Read the model definition and answer for the solid it produces. Units are mm, in the model's axes. Give positions to 0.01 mm unless a question says otherwise; leave off trailing zeros. Write each loop counter-clockwise with the first axis right and the second up, starting at its lowest first coordinate (ties: lowest second). Pieces come first, ordered by that corner, then holes. Notation, with made-up numbers: (17.5, 54) -> (38.5, 54) arc R8 ccw to (38.5, 65) -> close; hole circle Ø1 at (40, -4). An arc over 180 degrees is marked (long way). Answer as CSV lines item,"result". Start each with the question number.
1. The part is cut by section B-B, the plane x = 47. Determine the outline of the cut face in (y, z), and give its area (3 significant figures).
2. The part is cut by section A-A, the plane z = -244. Determine the outline of the cut face in (x, y), and give its area (3 significant figures).
3. The part is cut by section C-C, the plane x = 257. Determine the outline of the cut face in (y, z).
4. Find the intervals of material crossed by line 1 (X direction, y = 3.25, z = -40); line 2 (Z direction, x = 102.5, y = 2.5); line 3 (Z direction, x = 187, y = 3.25), in increasing order.
5. The part is cut by section D-D, the plane y = 4. Give the number of separate pieces and of enclosed holes in the cut face, and give its area (3 significant figures).
6. Given pin 1 (1.8 mm diameter, centred on x = 144.5, y = 2, fed in from -Z); pin 2 (1.5 mm diameter, centred on x = 162.5, y = 2.5, fed in from -Z); pin 3 (1.8 mm diameter, centred on x = 153.5, y = 2.5, fed in from +Z), each flat-ended and moving along its own axis, determine where each tip first touches the part or whether it passes through.
from build123d import *

# Parameters (mm, degrees)
SUPPORT_DEPTH = 6
SKETCH2_W     = 60
SKETCH2_H     = 100
LITE_DEPTH    = 468.118828565
FILLET1_R     = 1
FILLET2_R     = 1
SKETCH3_W     = 6
SKETCH3_H     = 40
SKETCH3_W_2   = 40
SKETCH3_H_2   = 6
MOUNT_DEPTH   = 468.118828565


with BuildPart() as part:
    # Sketch1 → support (new body)
    with BuildSketch(Plane(origin=(0, 0, 0), x_dir=(1, 0, 0), z_dir=(0, 1, 0))):
        Polygon((300, 0), (300, -12), (180, -70), (174, -70), (0, -6), (0, 0), (0, 288), (0, 294), (174, 358), (180, 358), (300, 300), (300, 288), align=None)
    extrude(amount=SUPPORT_DEPTH)

    # Sketch2 → lite (cut, through all)
    with BuildSketch(Plane(origin=(0, 6, 0), x_dir=(1, 0, 0), z_dir=(0, 1, 0))):
        Polygon((95.999022376, -20), (164.988314579, -20), (164.988314579, -45.375371845), align=None)
        Polygon((184.988314579, -20), (184.988314579, -45.375371845), (237.489083913, -20), align=None)
        Polygon((95.999022376, 308), (164.988314579, 333.375371845), (164.988314579, 308), align=None)
        Polygon((184.988314579, 333.375371845), (237.489083913, 308), (184.988314579, 308), align=None)
        with Locations((245, 64)):
            Rectangle(SKETCH2_W, SKETCH2_H)
        with Locations((150, 64)):
            Rectangle(SKETCH2_W, SKETCH2_H)
        with Locations((55, 64)):
            Rectangle(SKETCH2_W, SKETCH2_H)
        with Locations((55, 224)):
            Rectangle(SKETCH2_W, SKETCH2_H)
        with Locations((150, 224)):
            Rectangle(SKETCH2_W, SKETCH2_H)
        with Locations((245, 224)):
            Rectangle(SKETCH2_W, SKETCH2_H)
    extrude(amount=-LITE_DEPTH, mode=Mode.SUBTRACT)

    # Fillet1
    fillet1_edges = [part.edges().sort_by_distance(p)[0] for p in [
        (0, 3, -294),
        (174, 3, -358),
        (180, 3, -358),
        (300, 3, -300),
        (300, 3, 12),
        (180, 3, 70),
        (174, 3, 70),
        (0, 3, 6),
    ]]
    fillet(fillet1_edges, radius=FILLET1_R)

    # Fillet2
    fillet2_edges = [part.edges().sort_by_distance(p)[0] for p in [
        (85, 3, -114),
        (85, 3, -14),
        (25, 3, -14),
        (25, 3, -114),
        (85, 3, -274),
        (85, 3, -174),
        (25, 3, -174),
        (25, 3, -274),
        (180, 3, -274),
        (180, 3, -174),
        (120, 3, -174),
        (120, 3, -274),
        (275, 3, -274),
        (275, 3, -174),
        (215, 3, -174),
        (215, 3, -274),
        (164.988314579, 3, 45.375371845),
        (95.999022376, 3, 20),
        (164.988314579, 3, 20),
        (184.988314579, 3, 20),
        (237.489083913, 3, 20),
        (184.988314579, 3, 45.375371845),
        (164.988314579, 3, -308),
        (95.999022376, 3, -308),
        (164.988314579, 3, -333.375371845),
        (184.988314579, 3, -308),
        (184.988314579, 3, -333.375371845),
        (237.489083913, 3, -308),
        (275, 3, -114),
        (275, 3, -14),
        (215, 3, -14),
        (215, 3, -114),
        (180, 3, -114),
        (180, 3, -14),
        (120, 3, -14),
        (120, 3, -114),
    ]]
    fillet(fillet2_edges, radius=FILLET2_R)

    # Sketch3 → mount (cut, through all)
    with BuildSketch(Plane(origin=(0, 6, 0), x_dir=(1, 0, 0), z_dir=(0, 1, 0))):
        with Locations((3, 144)):
            Rectangle(SKETCH3_W, SKETCH3_H)
        with Locations((297, 144)):
            Rectangle(SKETCH3_W, SKETCH3_H)
        with Locations((170, -9.273001814)):
            Rectangle(SKETCH3_W_2, SKETCH3_H_2)
        with Locations((170, 296.372652861)):
            Rectangle(SKETCH3_W_2, SKETCH3_H_2)
    extrude(amount=-MOUNT_DEPTH, mode=Mode.SUBTRACT)


solid = part.part
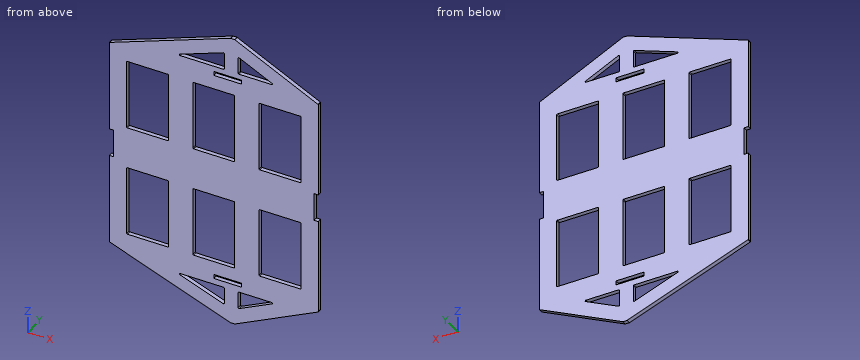
Results found:
1,outline,"(0, -311.29) -> (6, -311.29) -> (6, -274) -> (0, -274) -> close; (0, -174) -> (6, -174) -> (6, -114) -> (0, -114) -> close; (0, -14) -> (6, -14) -> (6, 23.29) -> (0, 23.29) -> close"
1,area,"807 mm²"
2,outline,"(0, 0) -> (25, 0) -> (25, 6) -> (0, 6) -> close; (85, 0) -> (120, 0) -> (120, 6) -> (85, 6) -> close; (180, 0) -> (215, 0) -> (215, 6) -> (180, 6) -> close; (275, 0) -> (300, 0) -> (300, 6) -> (275, 6) -> close"
2,area,"720 mm²"
3,outline,"(0, -320.78) -> (6, -320.78) -> (6, -274) -> (0, -274) -> close; (0, -174) -> (6, -174) -> (6, -114) -> (0, -114) -> close; (0, -14) -> (6, -14) -> (6, 32.78) -> (0, 32.78) -> close"
4,line 1,"x = 0 to 25, 85 to 120, 180 to 215, 275 to 300"
4,line 2,"z = -331.7 to -310.39, -308 to 20, 22.39 to 43.7"
4,line 3,"z = -354.62 to -332.4, -308 to -299.37, -293.37 to 6.27, 12.27 to 20, 44.4 to 66.62"
5,separate pieces,"1"
5,enclosed holes,"12"
5,area,"70,300 mm²"
6,pin 1,"stops at z = -347.48"
6,pin 2,"stops at z = -354.05"
6,pin 3,"stops at z = 62.79"
